Verification items for the finished model (mm, model axes). Give positions to 0.01 mm unless a question says otherwise; leave off trailing zeros. Order: outer loops, then holes, each group sorted by start corner. A loop starts at its lowest first (then second) coordinate and runs counter-clockwise, first axis right, second up.
from build123d import *

# Parameters (mm, degrees)
SKETCH_1_W          = 21
SKETCH_1_H          = 92
EXTRUDE_1_DEPTH     = 5
SKETCH_3_R          = 2.5
CUT_EXTRUDE_1_DEPTH = 15
SKETCH_4_R          = 2.5
CUT_EXTRUDE_2_DEPTH = 15
FILLET_2_R          = 10.5


with BuildPart() as part:
    # 草图1 → 凸台-拉伸1 (new body)
    with BuildSketch(Plane.XY):
        with Locations((-49.157142857, -8.885714286)):
            Rectangle(SKETCH_1_W, SKETCH_1_H)
    extrude(amount=EXTRUDE_1_DEPTH)

    # 草图3 → 切除-拉伸1 (cut)
    with BuildSketch(Plane.XY.offset(5)):
        with Locations((-49.157142857, -44.885714286)):
            Circle(SKETCH_3_R)
    extrude(amount=-CUT_EXTRUDE_1_DEPTH, mode=Mode.SUBTRACT)

    # 草图4 → 切除-拉伸2 (cut)
    with BuildSketch(Plane.XY.offset(5)):
        with Locations((-49.157142857, 27.114285714)):
            Circle(SKETCH_4_R)
    extrude(amount=-CUT_EXTRUDE_2_DEPTH, mode=Mode.SUBTRACT)

    # 圆角2
    fillet_2_edges = [part.edges().sort_by_distance(p)[0] for p in [
        (-38.657142857, 37.114285714, 2.5),
        (-59.657142857, 37.114285714, 2.5),
        (-38.657142857, -54.885714286, 2.5),
        (-59.657142857, -54.885714286, 2.5),
    ]]
    fillet(fillet_2_edges, radius=FILLET_2_R - 0.0001)  # a hair under: the kernel refuses the full size


solid = part.part
(1) Section check C-C, the plane y = 30.5. Enter the section's corners in (x, z).
Solved:
outline: (-58.91, 0) - (-39.4, 0) - (-39.4, 5) - (-58.91, 5) - close
(2) Section check D-D, the plane x = -41.75. Enter the section's corners in (y, z).
Solved:
outline: (-51.83, 0) - (34.06, 0) - (34.06, 5) - (-51.83, 5) - close
(3) Section check B-B, the plane z = 2.1. Give the number of separate pieces and of enclosed holes in the cut face, then the cut area to 3 significant figures.
Solved:
separate pieces: 1
enclosed holes: 2
area: 1,800 mm2
(4) Go/stop test with flat-tipped pins: pin 1 (5 mm diameter, centred on x = -55.5, y = -7.5, fed in from -Z); pin 2 (4 mm diameter, centred on x = -49.16, y = 27.11, fed in from -Z). Record where each tip stops, or that it passes through.
Solved:
pin 1: stops at z = 0
pin 2: passes through
(5) Scan lines: line 1 (X direction, y = 27, z = 2.5); line 2 (Y direction, x = -50, z = 0.35); line 3 (Y direction, x = -41.5, z = 0.45). Record each from-to range of solid material in increasing order.
Solved:
line 1: x = -59.65 to -51.65, -46.66 to -38.66
line 2: y = -54.85 to -47.24, -42.53 to 24.76, 29.47 to 37.08
line 3: y = -51.57 to 33.8
(6) Release check for a two-part mould opening along X. For faces 1 (the flat face through (-49, -8, 0)), 2 (the cylindrical face through (-41.815, -51.892, 2.535)), 3 (the cylindrical face through (-49.699, 24.674, 2.535)) record: pulls with the +X half, pulls with the -X half, needs draft (parallel to the pull), parting line crosses it, or undercut.
Solved:
face 1: needs draft
face 2: pulls with the +X half
face 3: undercut
(7) Section check A-A, the plane x = -47.5. Enter the section's corners in (y, z).
Solved:
outline: (-54.75, 0) - (-46.76, 0) - (-46.76, 5) - (-54.75, 5) - close; (-43.01, 0) - (25.24, 0) - (25.24, 5) - (-43.01, 5) - close; (28.99, 0) - (36.98, 0) - (36.98, 5) - (28.99, 5) - close
